```python
from build123d import *

# Parameters (mm, degrees)
SKETCH1_R               = 9.5
BOSS_EXTRUDE1_DEPTH     = 20
SKETCH2_R               = 4.75
BOSS_EXTRUDE2_DEPTH     = 3.5
SKETCH3_R               = 6.5
BOSS_EXTRUDE3_DEPTH     = 9.5
SKETCH4_R               = 8
BOSS_EXTRUDE4_DEPTH     = 100.5
SKETCH5_R               = 6.5
BOSS_EXTRUDE5_DEPTH     = 6.5
SKETCH6_R               = 9.5
BOSS_EXTRUDE6_DEPTH     = 20
CUT_EXTRUDE1_DEPTH      = 161.563071719
CUT_EXTRUDE1_DEPTH_BACK = 161.563071719
SKETCH7_R               = 4.1
FILLET1_R               = 1.5


with BuildPart() as part:
    # Sketch1 → Boss-Extrude1 (new body)
    with BuildSketch(Plane.XY):
        Circle(SKETCH1_R)
    extrude(amount=BOSS_EXTRUDE1_DEPTH)

    # Sketch2 → Boss-Extrude2 (add)
    with BuildSketch(Plane.XY.offset(20)):
        Circle(SKETCH2_R)
    extrude(amount=BOSS_EXTRUDE2_DEPTH)

    # Sketch3 → Boss-Extrude3 (add)
    with BuildSketch(Plane.XY.offset(23.5)):
        Circle(SKETCH3_R)
    extrude(amount=BOSS_EXTRUDE3_DEPTH)

    # Sketch4 → Boss-Extrude4 (add)
    with BuildSketch(Plane.XY.offset(33)):
        Circle(SKETCH4_R)
    extrude(amount=BOSS_EXTRUDE4_DEPTH)

    # Sketch5 → Boss-Extrude5 (add)
    with BuildSketch(Plane.XY.offset(133.5)):
        Circle(SKETCH5_R)
    extrude(amount=BOSS_EXTRUDE5_DEPTH)

    # Sketch6 → Boss-Extrude6 (add)
    with BuildSketch(Plane.XY.offset(140)):
        Circle(SKETCH6_R)
    extrude(amount=BOSS_EXTRUDE6_DEPTH)

    # Sketch7 → Cut-Extrude1 (cut, two sides: drawn at the far end of the back side and taken through both)
    with BuildSketch(Plane(origin=(0, 0, 0), x_dir=(0, 0, -1), z_dir=(1, 0, 0)).offset(-CUT_EXTRUDE1_DEPTH_BACK)):
        with Locations((-150, -0.5)):
            Circle(SKETCH7_R)
    extrude(amount=CUT_EXTRUDE1_DEPTH + CUT_EXTRUDE1_DEPTH_BACK, mode=Mode.SUBTRACT)

    # Fillet1
    fillet1_edges = [part.edges().sort_by_distance(p)[0] for p in [
        (-9.5, 0, 160),
    ]]
    fillet(fillet1_edges, radius=FILLET1_R)


solid = part.part
```
Build history of the part. All positions in model axes, mm. A direction names the side the tool comes from. Give positions to 0.01 mm unless a question says otherwise; leave off trailing zeros. Loops run counter-clockwise (first coordinate to the right, second up) from the corner with the lowest first, then second, coordinate; pieces in that order, holes last.
Item 1: Slice it at A-A, the plane x = 0. List the corners of the cut face in (y, z), and give its area (3 significant figures).
Answers follow:
outline: (-9.5, 0) - (9.5, 0) - (9.5, 20) - (4.75, 20) - (4.75, 23.5) - (6.5, 23.5) - (6.5, 33) - (8, 33) - (8, 133.5) - (6.5, 133.5) - (6.5, 140) - (9.5, 140) - (9.5, 158.5) arc R1.5 ccw to (8, 160) - (-8, 160) arc R1.5 ccw to (-9.5, 158.5) - (-9.5, 140) - (-6.5, 140) - (-6.5, 133.5) - (-8, 133.5) - (-8, 33) - (-6.5, 33) - (-6.5, 23.5) - (-4.75, 23.5) - (-4.75, 20) - (-9.5, 20) - close; hole circle Ø8.2 at (-0.5, 150)
area: 2,560 mm2
Item 2: Pull direction Z, two halves, no side cores. Call faces 3 (the face through (0, -5, 23.5)), 4 (the face through (4, -6, 140)), 5 (the face through (4.38, -8.43, 9.86)), 6 (the face through (0, 0, 160)): released by +Z, released by -Z, zero draft, split by the parting line, or undercut.
Answers follow:
face 3: undercut
face 4: undercut
face 5: zero draft
face 6: released by +Z
Item 3: Slice it at B-B, the plane z = 28. List the corners of the cut face in (x, y).
Answers follow:
outline: circle Ø13 at (0, 0)
Item 4: Flat gauge pins, fed straight in: pin 1 (3 mm diameter, centred on y = -1, z = 127.5, fed in from +X); pin 2 (5 mm diameter, centred on y = 6, z = 118.5, fed in from +X); pin 3 (8 mm diameter, centred on y = 3.5, z = 31, fed in from -X). Where does each tip first touch, or does it go through?
Answers follow:
pin 1: stops at x = 8
pin 2: stops at x = 7.19
pin 3: stops at x = -8
Item 5: Slice it at C-C, the plane z = 149. List the corners of the cut face in (x, y), and give its area (3 significant figures).
Answers follow:
outline: (-8.84, 3.48) - (8.84, 3.48) arc R9.5 ccw to start; (-8.38, -4.48) arc R9.5 ccw to (8.38, -4.48) - close
area: 137 mm2
Item 6: Drill centre lines: line 1 (Z direction, x = -1, y = -7.75); line 2 (Z direction, x = 3.25, y = -0.5); line 3 (Z direction, x = -4.75, y = 4.25). Where is each one in solid material? Low to high.
Answers follow:
line 1: z = 0 to 20, 33 to 133.5, 140 to 160
line 2: z = 0 to 145.9, 154.1 to 160
line 3: z = 0 to 20, 23.5 to 160
Item 7: Which spindle directions (+Z, -Z, +X, -X, +Y, -Y) get a long thin tool onto all of the face, cutting with end or side? Do faces 1 (the face through (-0.135, 3.565, 150.534)), 2 (the face through (-1.73, -7.81, 82.55)). Say none if no direction does.
Answers follow:
face 1: +X, -X
face 2: none
